```python
from build123d import *

# Parameters (mm, degrees)
F0_R     = 4.05
F1_DEPTH = 20
F2_W     = 2
F2_H     = 25.5416983529
F3_DEPTH = 25
F4_R     = 3
F5_DEPTH = 25
F6_R     = 3
F7_DEPTH = 25
F8_R     = 5
F9_R     = 1


with BuildPart() as f1:
    # F0 (on Top) → F1 (new body)
    with BuildSketch(Plane.XY):
        Polygon((6, 28), (0, 28), (-6, 28), (-6, 4), (-18, 4), (-18, 0), (0, 0), (18, 0), (18, 4), (6, 4), align=None)
        with Locations((0, 10)):
            Circle(F0_R, mode=Mode.SUBTRACT)
    extrude(amount=F1_DEPTH)

    # F2 (on face) → F3 (cut)
    with BuildSketch(Plane.XY.offset(20)):
        with Locations((0, 21.3338027536)):
            Rectangle(F2_W, F2_H)
    extrude(amount=-F3_DEPTH, mode=Mode.SUBTRACT)

    # F4 (on face) → F5 (cut)
    with BuildSketch(Plane(origin=(-6, 0, 0), x_dir=(0, -1, 0), z_dir=(-1, 0, 0))):
        with Locations((-20, 9.9280960858)):
            Circle(F4_R)
    extrude(amount=-F5_DEPTH, mode=Mode.SUBTRACT)

    # F6 (on face) → F7 (cut)
    with BuildSketch(Plane(origin=(0, 4, 0), x_dir=(-1, 0, 0), z_dir=(0, 1, 0))):
        with Locations((12, 10)):
            Circle(F6_R)
        with Locations((-12, 10)):
            Circle(F6_R)
    extrude(amount=-F7_DEPTH, mode=Mode.SUBTRACT)

    # F8
    f8_edges = [f1.edges().sort_by_distance(p)[0] for p in [
        (3.5, 28, 20),
        (-3.5, 28, 20),
        (-18, 2, 20),
        (18, 2, 20),
    ]]
    fillet(f8_edges, radius=F8_R)

    # F9
    f9_edges = [f1.edges().sort_by_distance(p)[0] for p in [
        (0, 5.95, 20),
        (-9, 4, 10),
        (15, 4, 10),
        (-6, 23, 9.928096),
        (6, 23, 9.928096),
    ]]
    fillet(f9_edges, radius=F9_R)


solid = f1.part
```
The listing builds one solid part. Answer for the finished solid, in the listing's coordinates (mm). A direction names the side the tool comes from. Coordinates: 2 decimals unless noted, no trailing zeros. Write each loop counter-clockwise with the first axis right and the second up, starting at its lowest first coordinate (ties: lowest second). Pieces come first, ordered by that corner, then holes. Notation, with made-up numbers: (89, 88) - (148, 88) arc R17 cw to (148, 103) - close; hole circle Ø9 at (-10, 35.5). An arc over 180 degrees is marked (long way). Return JSON: item names as keys, results as strings. Group by question number.
1. A cutting plane is placed at A-A, the plane x = -12. Determine the outline of the cut face in (y, z).
2. A cutting plane is placed at D-D, the plane x = 0. Determine the outline of the cut face in (y, z), plus the area to 3 significant figures.
3. Given pin 1 (1.5 mm diameter, centred on y = 24, z = 15.5, fed in from -X); pin 2 (7 mm diameter, centred on x = 12, z = 10, fed in from +Y); pin 3 (9.5 mm diameter, centred on x = 11.5, z = 13, fed in from +Y); pin 4 (5 mm diameter, centred on x = -12, z = 10, fed in from -Y), each flat-ended and moving along its own axis, determine where each tip first touches the part or whether it passes through.
4. Determine the mould class of faces 1 (the cylindrical face through (2.972, 22.211, 11.956)), 2 (the flat face through (1, 22.43, 7.92)), 3 (the flat face through (4, 28, 7)) for opening direction Y: released by +Y, released by -Y, zero draft, split by the parting line, or undercut.
5. Straight lines are drawn through the part: L1, parallel to X at y = 27, z = 14.25; L2, parallel to Z at x = 12, y = 1.8; L3, parallel to Z at x = 2.2, y = 20. For each, find the intervals that lie inside material, in ascending order.
6. Which of the six approach directions +Z, -Z, +X, -X, +Y, -Y give full straight-line access (tool end or side, diameter ignored) to faces 4 (the flat face through (-6, 16, 8)), 5 (the flat face through (12, 4, 5)), 6 (the cylindrical face through (-3.028, 22.211, 11.956)), 7 (the flat face through (-1, 22.43, 7.92)), 8 (the flat face through (-3.1, 14.2, 20))?
7. A cutting plane is placed at C-C, the plane y = 10. Determine the outline of the cut face in (x, z).
8. A cutting plane is placed at B-B, the plane z = 2.5. Determine the outline of the cut face in (x, y), plus the area to 3 significant figures.
Ans:
{
 "1": {"outline": "(0, 0) - (4, 0) - (4, 6) arc R1 ccw to (3, 7) - (0, 7) - close; (0, 13) - (3, 13) arc R1 ccw to (4, 14) - (4, 20) - (0, 20) - close"},
 "2": {"outline": "(0, 0) - (5.95, 0) - (5.95, 19) arc R1 ccw to (4.95, 20) - (0, 20) - close", "area": "119 mm²"},
 "3": {"pin 1": "x = -6", "pin 2": "y = 3.87", "pin 3": "y = 4", "pin 4": "through"},
 "4": {"face 1": "undercut", "face 2": "zero draft", "face 3": "released by +Y"},
 "5": {"L1": "-6 to -1, 1 to 6", "L2": "0 to 7, 13 to 20", "L3": "0 to 6.93, 12.93 to 20"},
 "6": {"face 4": "+Z, -Z, -X, +Y", "face 5": "+Z, -Z, +X, +Y", "face 6": "+X, -X", "face 7": "+Z, -Z, +Y", "face 8": "+Z, +X, -X, +Y, -Y"},
 "7": {"outline": "(-6, 0) - (-4.05, 0) - (-4.05, 19) arc R1 ccw to (-5.05, 20) - (-6, 20) - close; (4.05, 0) - (6, 0) - (6, 20) - (5.05, 20) arc R1 ccw to (4.05, 19) - close"},
 "8": {"outline": "(-18, 0) - (18, 0) - (18, 4) - (6, 4) - (6, 28) - (1, 28) - (1, 13.92) arc R4.05 cw (long way) to (-1, 13.92) - (-1, 28) - (-6, 28) - (-6, 4) - (-18, 4) - close", "area": "352 mm²"}
}
